from build123d import *

# Parameters (mm, degrees)
SKETCH1_R           = 45
SKETCH1_R_2         = 8
SKETCH1_R_3         = 1.55
BOSS_EXTRUDE1_DEPTH = 10


with BuildPart() as part:
    # Sketch1 → Boss-Extrude1 (new body)
    # profile 1 of 2: a face of its own
    with BuildSketch(Plane(origin=(0, 0, 0), x_dir=(1, 0, 0), z_dir=(0, 1, 0))):
        with Locations(Location((0, 0, 0), (0, 0, 270))):
            Circle(SKETCH1_R)
        with BuildLine():
            Line((0, 8), (0, 40))
            ThreePointArc((0, 40), (8.657584558, 39.051840285), (16.90473047, 36.252311481))
            Line((16.90473047, 36.252311481), (3.380946094, 7.250462296))
            ThreePointArc((3.380946094, 7.250462296), (4.588611491, 6.553216354), (5.656854249, 5.656854249))
            Line((5.656854249, 5.656854249), (28.284271247, 28.284271247))
            ThreePointArc((28.284271247, 28.284271247), (33.735657833, 21.491984334), (37.587704831, 13.680805733))
            Line((37.587704831, 13.680805733), (7.517540966, 2.736161147))
            ThreePointArc((7.517540966, 2.736161147), (7.878462024, 1.389185421), (8, 0))
            Line((8, 0), (40, 0))
            ThreePointArc((40, 0), (39.051840285, -8.657584558), (36.252311481, -16.90473047))
            Line((36.252311481, -16.90473047), (7.250462296, -3.380946094))
            ThreePointArc((7.250462296, -3.380946094), (6.553216354, -4.588611491), (5.656854249, -5.656854249))
            Line((5.656854249, -5.656854249), (28.284271247, -28.284271247))
            ThreePointArc((28.284271247, -28.284271247), (21.491984334, -33.735657833), (13.680805733, -37.587704831))
            Line((13.680805733, -37.587704831), (2.736161147, -7.517540966))
            ThreePointArc((2.736161147, -7.517540966), (1.389185421, -7.878462024), (0, -8))
            Line((0, -8), (0, -40))
            ThreePointArc((0, -40), (-8.657584558, -39.051840285), (-16.90473047, -36.252311481))
            Line((-16.90473047, -36.252311481), (-3.380946094, -7.250462296))
            ThreePointArc((-3.380946094, -7.250462296), (-4.588611491, -6.553216354), (-5.656854249, -5.656854249))
            Line((-5.656854249, -5.656854249), (-28.284271247, -28.284271247))
            ThreePointArc((-28.284271247, -28.284271247), (-33.735657833, -21.491984334), (-37.587704831, -13.680805733))
            Line((-37.587704831, -13.680805733), (-7.517540966, -2.736161147))
            ThreePointArc((-7.517540966, -2.736161147), (-7.878462024, -1.389185421), (-8, 0))
            Line((-8, 0), (-40, 0))
            ThreePointArc((-40, 0), (-39.051840285, 8.657584558), (-36.252311481, 16.90473047))
            Line((-36.252311481, 16.90473047), (-7.250462296, 3.380946094))
            ThreePointArc((-7.250462296, 3.380946094), (-6.553216354, 4.588611491), (-5.656854249, 5.656854249))
            Line((-5.656854249, 5.656854249), (-28.284271247, 28.284271247))
            ThreePointArc((-28.284271247, 28.284271247), (-21.491984334, 33.735657833), (-13.680805733, 37.587704831))
            Line((-13.680805733, 37.587704831), (-2.736161147, 7.517540966))
            ThreePointArc((-2.736161147, 7.517540966), (-1.389185421, 7.878462024), (0, 8))
        make_face(mode=Mode.SUBTRACT)
    # profile 2 of 2: a face of its own
    with BuildSketch(Plane(origin=(0, 0, 0), x_dir=(1, 0, 0), z_dir=(0, 1, 0))):
        Circle(SKETCH1_R_2)
        with Locations(Location((0, 0, 0), (0, 0, 270))):
            Circle(SKETCH1_R_3, mode=Mode.SUBTRACT)
    extrude(amount=BOSS_EXTRUDE1_DEPTH)


solid = part.part
Build history of the part. All positions in model axes, mm. A direction names the side the tool comes from. Coordinates: 2 decimals unless noted, no trailing zeros. Order: outer loops, then holes, each group sorted by start corner. A loop starts at its lowest first (then second) coordinate and runs counter-clockwise, first axis right, second up. Notation, with made-up numbers: (-39, -4.5) - (-8, -4.5) arc R34 ccw to (-8, 33.5) - close; hole circle Ø3 at (73, 70). An arc over 180 degrees is marked (long way). Write item = value, one per line. Start each with the question number.
1) Saw through at A-A on y = 4.75. Count the separate pieces of the cut face and the enclosed holes in it, then the cut area to 3 significant figures.
2) Saw through at B-B on z = 12. Write the cut outline in (x, y), then the cut area to 3 significant figures.
3) Saw through at C-C on x = -33.5. Write the cut outline in (y, z), then the cut area to 3 significant figures.
4) Flat gauge pins, fed straight in: pin 1 Ø2.5 at (x, z) = (0, 0) entering from -Y; pin 2 Ø4 at (x, y) = (7.5, 6.5) entering from +Z; pin 3 Ø5 at (x, y) = (-19.5, 6.5) entering from -Z; pin 4 Ø1 at (x, y) = (26.5, 3.5) entering from +Z. Where does each tip first touch, or does it go through?
5) 3-axis set-ups, long thin cutter, end or side, ignore diameter. For faces 1 (the face through (9, 10, -1)), 2 (the face through (-10.238, 4.93, 21.954)): which of +Z, -Z, +X, -X, +Y, -Y reach the whole face in a straight line?
6) Wall check: line 1 along X through (y, z) = (9.75, 34); line 2 along X through (y, z) = (8, -21); line 3 along Z through (x, y) = (-19.5, 7.5). Give the ranges that are in metal, low to high. Write a range as from..to.
7) Two-plate mould, pull along Z, no slides. Class faces 3 (the face through (9, 0, -1)), 4 (the face through (-8.538, 4.93, 39.078)): pulls with the +Z half, pulls with the -Z half, needs draft (parallel to the pull), parting line crosses it, or undercut.
From the geometry:
q1.separate_pieces = 1
q1.enclosed_holes = 9
q1.area = 3,670 mm^2
q2.outline = (-43.37, 0) - (-32.97, 0) - (-32.97, 10) - (-43.37, 10) - close; (-12, 0) - (-5.6, 0) - (-5.6, 10) - (-12, 10) - close; (0, 0) - (4.37, 0) - (4.37, 10) - (0, 10) - close; (12, 0) - (25.73, 0) - (25.73, 10) - (12, 10) - close; (38.16, 0) - (43.37, 0) - (43.37, 10) - (38.16, 10) - close
q2.area = 401 mm^2
q3.outline = (0, -30.05) - (10, -30.05) - (10, -15.62) - (0, -15.62) - close; (0, 0) - (10, 0) - (10, 12.19) - (0, 12.19) - close; (0, 21.86) - (10, 21.86) - (10, 30.05) - (0, 30.05) - close
q3.area = 348 mm^2
q4.pin_1 = through
q4.pin_2 = 44.66
q4.pin_3 = -41.67
q4.pin_4 = 36.73
q5.face_1 = +Z, -Z, +X, -X, +Y
q5.face_2 = +Y, -Y
q6.line_1 = -29.48..-15.85, 0..12.37, 21.07..29.48
q6.line_2 = -39.8..-21, -7.64..0, 9.79..21, 34.04..39.8
q6.line_3 = -40.56..-34.92, -19.5..-9.09, 0..7.1, 19.5..40.56
q7.face_3 = needs draft
q7.face_4 = undercut
